Build history of the part. All positions in model axes, mm. Face numbers are marked on the shaded views. Give positions to 0.01 mm unless a question says otherwise; leave off trailing zeros. Write each loop counter-clockwise with the first axis right and the second up, starting at its lowest first coordinate (ties: lowest second). Pieces come first, ordered by that corner, then holes. Notation, with made-up numbers: M 69.25,-24.75 L 115.25,-24.75 A18 cw 115.25,6.25 Z; hole C -12,24 d6. An arc over 180 degrees is marked long. One line per item, written item: value. Start each with the question number.
from build123d import *

# Parameters (mm, degrees)
F1_DEPTH = 3.2
F2_DEPTH = 1.6
F3_DEPTH = 2.5


with BuildPart() as f1:
    # F0 (on Top) → F1 (new body)
    with BuildSketch(Plane.XY):
        with BuildLine():
            Line((5.7308066454, 15.4116954654), (9.2615315623, 22.3554545173))
            ThreePointArc((9.2615315623, 22.3554545173), (6.124599836, 23.4100745493), (2.8731075212, 24.026809333))
            Line((2.8731075212, 24.026809333), (-12.0286401361, 7.7058477327))
            Line((-12.0286401361, 7.7058477327), (-2.0674222615, 7.7058477327))
            Line((-2.0674222615, 7.7058477327), (-18.230907619, -9.2094279826))
            Line((-18.230907619, -9.2094279826), (-4.3697794008, -9.2094279826))
            Line((-4.3697794008, -9.2094279826), (-11.0294978873, -21.5381635686))
            ThreePointArc((-11.0294978873, -21.5381635686), (-8.7153894779, -22.573973948), (-6.3056047528, -23.3619704275))
            Line((-6.3056047528, -23.3619704275), (10.7070716166, -3.7589499261))
            Line((10.7070716166, -3.7589499261), (1.6710584512, -3.7589499261))
            Line((1.6710584512, -3.7589499261), (15.9755367786, 15.4116954654))
            Line((15.9755367786, 15.4116954654), (5.7308066454, 15.4116954654))
        make_face()
        with BuildLine():
            Line((-7.468564605, -24.7020021385), (-6.3056047528, -23.3619704275))
            ThreePointArc((-6.3056047528, -23.3619704275), (-8.7153894779, -22.573973948), (-11.0294978873, -21.5381635686))
            Line((-11.0294978873, -21.5381635686), (-11.7940875977, -22.9536024329))
            ThreePointArc((-11.7940875977, -22.9536024329), (-9.6709186664, -23.9257538869), (-7.468564605, -24.7020021385))
        make_face()
        with BuildLine():
            ThreePointArc((2.8731075212, 24.026809333), (6.124599836, 23.4100745493), (9.2615315623, 22.3554545173))
            Line((9.2615315623, 22.3554545173), (9.9925901152, 23.7932030147))
            ThreePointArc((9.9925901152, 23.7932030147), (7.1383273937, 24.799448561), (4.1858882241, 25.464616759))
            Line((4.1858882241, 25.464616759), (2.8731075212, 24.026809333))
        make_face()
        with BuildLine():
            ThreePointArc((4.1858882241, 25.464616759), (7.1383273937, 24.799448561), (9.9925901152, 23.7932030147))
            Line((9.9925901152, 23.7932030147), (19.2086462315, 41.9181135037))
            Line((19.2086462315, 41.9181135037), (4.1858882241, 25.464616759))
        make_face()
        with BuildLine():
            Line((-21.4260146022, -40.7846085727), (-7.468564605, -24.7020021385))
            ThreePointArc((-7.468564605, -24.7020021385), (-9.6709186664, -23.9257538869), (-11.7940875977, -22.9536024329))
            Line((-11.7940875977, -22.9536024329), (-21.4260146022, -40.7846085727))
        make_face()
    extrude(amount=F1_DEPTH)

    # F0 (on Top) → F2 (join)
    with BuildSketch(Plane.XY):
        with BuildLine():
            ThreePointArc((-6.3056047528, -23.3619704275), (14.7132492292, -19.2110023339), (24.1979816008, 0))
            ThreePointArc((24.1979816008, 0), (20.1202967659, 13.4430640706), (9.2615315623, 22.3554545173))
            Line((9.2615315623, 22.3554545173), (5.7308066454, 15.4116954654))
            Line((5.7308066454, 15.4116954654), (15.9755367786, 15.4116954654))
            Line((15.9755367786, 15.4116954654), (1.6710584512, -3.7589499261))
            Line((1.6710584512, -3.7589499261), (10.7070716166, -3.7589499261))
            Line((10.7070716166, -3.7589499261), (-6.3056047528, -23.3619704275))
        make_face()
        with BuildLine():
            Line((-12.0286401361, 7.7058477327), (2.8731075212, 24.026809333))
            ThreePointArc((2.8731075212, 24.026809333), (-23.1446184854, 7.061795007), (-11.0294978873, -21.5381635686))
            Line((-11.0294978873, -21.5381635686), (-4.3697794008, -9.2094279826))
            Line((-4.3697794008, -9.2094279826), (-18.230907619, -9.2094279826))
            Line((-18.230907619, -9.2094279826), (-2.0674222615, 7.7058477327))
            Line((-2.0674222615, 7.7058477327), (-12.0286401361, 7.7058477327))
        make_face()
    extrude(amount=F2_DEPTH)

    # F0 (on Top) → F3 (join)
    with BuildSketch(Plane.XY):
        with BuildLine():
            ThreePointArc((-11.0294978873, -21.5381635686), (-23.1446184854, 7.061795007), (2.8731075212, 24.026809333))
            Line((2.8731075212, 24.026809333), (4.1858882241, 25.464616759))
            ThreePointArc((4.1858882241, 25.464616759), (-24.5061657926, 8.0880285022), (-11.7940875977, -22.9536024329))
            Line((-11.7940875977, -22.9536024329), (-11.0294978873, -21.5381635686))
        make_face()
        with BuildLine():
            ThreePointArc((9.2615315623, 22.3554545173), (20.1202967659, 13.4430640706), (24.1979816008, 0))
            ThreePointArc((24.1979816008, 0), (14.7132492292, -19.2110023339), (-6.3056047528, -23.3619704275))
            Line((-6.3056047528, -23.3619704275), (-7.468564605, -24.7020021385))
            ThreePointArc((-7.468564605, -24.7020021385), (15.3823255436, -20.7208211174), (25.8063629151, 0))
            ThreePointArc((25.8063629151, 0), (21.4923332131, 14.2845363931), (9.9925901152, 23.7932030147))
            Line((9.9925901152, 23.7932030147), (9.2615315623, 22.3554545173))
        make_face()
    extrude(amount=F3_DEPTH)


solid = f1.part
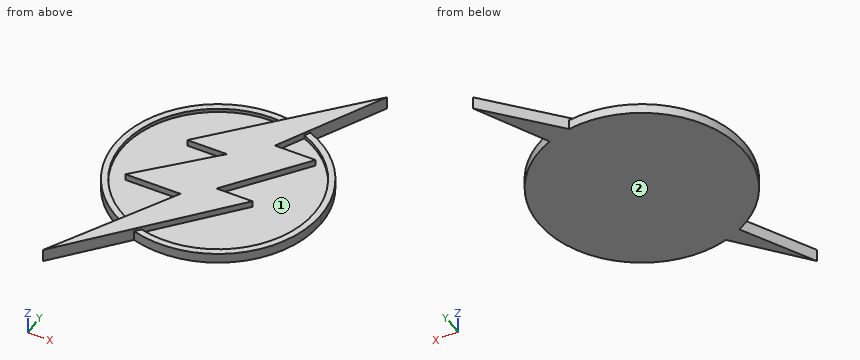
1) Probe line 1 along Y through (x, z) = (7, 2.7); line 2 along Y through (x, z) = (-11.5, 1.8); line 3 along X through (y, z) = (-13, 2.3). List the from-to ranges inside material, lowest first. Write a range as from..to.
2) Band-saw the part on B-B (x = -13). List the corners of the cut face in (y, z).
3) Band-saw the part on C-C (y = 16.5). List the corners of the cut face in (x, z), then the cut area to 3 significant figures.
4) Mould opens along Y. For the marked faces 1 and 2 say: released by +Y, released by -Y, zero draft, split by the parting line, or undercut.
5) Band-saw the part on D-D (x = 15). List the corners of the cut face in (y, z), then the cut area to 3 significant figures.
6) Band-saw the part on A-A (z = 0.95). List the corners of the cut face in (x, y).
7) Drop flat-ended pins along their axis: P1, Ø12, axis at x = 15.5, y = 10.5, coming from the +Z side; P2, Ø1.8, axis at x = -12, z = 2.5, coming from the -Y side; P3, Ø1.3, axis at x = -8, z = 2, coming from the -Y side; P4, Ø0.8, axis at x = 8.5, z = 2.5, coming from the +Y side. Give the stop position or say it passes through.
Model answer:
1. line 1: y = -8.03..-3.76, 3.38..15.41, 17.91..28.55
1. line 2: y = -29.35..-21.29, -9.21..-2.17, 7.71..8.28, 21.29..23.1
1. line 3: x = -22.29..-20.41, -6.42..2.69, 20.41..22.29
2. outline: M -31.08,0 L -25.19,0 L -25.19,3.2 L -31.08,3.2 Z; M -22.29,0 L 22.29,0 L 22.29,2.5 L 20.41,2.5 L 20.41,1.6 L -3.74,1.6 L -3.74,3.2 L -9.21,3.2 L -9.21,1.6 L -20.41,1.6 L -20.41,2.5 L -22.29,2.5 Z
3. outline: M -19.84,0 L 19.84,0 L 19.84,2.5 L 17.7,2.5 L 17.7,1.6 L 6.28,1.6 L 6.28,3.2 L -4,3.2 L -4,1.6 L -17.7,1.6 L -17.7,2.5 L -19.84,2.5 Z
3. area: 83.8 mm²
4. face 1: undercut
4. face 2: zero draft
5. outline: M -21,0 L 21,0 L 21,2.5 L 18.99,2.5 L 18.99,1.6 L 15.41,1.6 L 15.41,3.2 L 14.1,3.2 L 14.1,1.6 L -18.99,1.6 L -18.99,2.5 L -21,2.5 Z; M 33.64,0 L 37.31,0 L 37.31,3.2 L 33.64,3.2 Z
5. area: 84.6 mm²
6. outline: M -21.43,-40.78 L -7.47,-24.7 A25.81 ccw 9.99,23.79 L 19.21,41.92 L 4.19,25.46 A25.81 ccw -11.79,-22.95 Z
7. P1: stops at z = 3.2
7. P2: stops at y = -30.96
7. P3: stops at y = -26.06
7. P4: stops at y = 30.63
